```python
from build123d import *

# Parameters (mm, degrees)
SKETCH1_W           = 161.925
SKETCH1_H           = 152.4
SKETCH1_R           = 3.175
BOSS_EXTRUDE1_DEPTH = 12.7


with BuildPart() as part:
    # Sketch1 → Boss-Extrude1 (new body)
    with BuildSketch(Plane(origin=(0, 0, 0), x_dir=(0, 0, -1), z_dir=(1, 0, 0))):
        with Locations((20.6375, 0)):
            Rectangle(SKETCH1_W, SKETCH1_H)
        with Locations((95.25, -63.5)):
            Circle(SKETCH1_R, mode=Mode.SUBTRACT)
        with Locations((95.25, 0)):
            Circle(SKETCH1_R, mode=Mode.SUBTRACT)
        with Locations((-53.975, -63.5)):
            Circle(SKETCH1_R, mode=Mode.SUBTRACT)
        with Locations((-53.975, 0)):
            Circle(SKETCH1_R, mode=Mode.SUBTRACT)
        with Locations((95.25, 57.15)):
            Circle(SKETCH1_R, mode=Mode.SUBTRACT)
        with Locations((-53.975, 57.15)):
            Circle(SKETCH1_R, mode=Mode.SUBTRACT)
        with BuildLine():
            ThreePointArc((-33.455, 30.43), (-32.255, 29.23), (-33.455, 28.03))
            Line((-33.455, 28.03), (-36.055, 28.03))
            ThreePointArc((-36.055, 28.03), (-37.255, 29.23), (-36.055, 30.43))
            Line((-36.055, 30.43), (-33.455, 30.43))
        make_face(mode=Mode.SUBTRACT)
        with BuildLine():
            Line((-8.915, 28.03), (-11.515, 28.03))
            ThreePointArc((-11.515, 28.03), (-12.715, 29.23), (-11.515, 30.43))
            Line((-11.515, 30.43), (-8.915, 30.43))
            ThreePointArc((-8.915, 30.43), (-7.715, 29.23), (-8.915, 28.03))
        make_face(mode=Mode.SUBTRACT)
        with BuildLine():
            Line((-36.055, 48.17), (-33.455, 48.17))
            ThreePointArc((-33.455, 48.17), (-32.255, 46.97), (-33.455, 45.77))
            Line((-33.455, 45.77), (-36.055, 45.77))
            ThreePointArc((-36.055, 45.77), (-37.255, 46.97), (-36.055, 48.17))
        make_face(mode=Mode.SUBTRACT)
        with BuildLine():
            ThreePointArc((-8.915, 48.17), (-7.715, 46.97), (-8.915, 45.77))
            Line((-8.915, 45.77), (-11.515, 45.77))
            ThreePointArc((-11.515, 45.77), (-12.715, 46.97), (-11.515, 48.17))
            Line((-11.515, 48.17), (-8.915, 48.17))
        make_face(mode=Mode.SUBTRACT)
    extrude(amount=BOSS_EXTRUDE1_DEPTH)


solid = part.part
```
Design review of the part built by this model. Coordinates are the model's own, in mm. Coordinates: 2 decimals unless noted, no trailing zeros. Order: outer loops, then holes, each group sorted by start corner. A loop starts at its lowest first (then second) coordinate and runs counter-clockwise, first axis right, second up.
1) Take a section at A-A, the plane z = -95.25. Give the boundary of the cut face in (x, y) (3 decimals), and give its area (3 significant figures).
2) Take a section at B-B, the plane y = 57.15. Give the boundary of the cut face in (x, z) (3 decimals).
3) Wall thickness on line 1 along Y through (x, z) = (3.5, -95.25) (3 decimals): over which ranges is the line inside the solid? List them lowest first.
4) Clearance check with a flat-ended pin moving along its axis: pin 1 (5.5 mm diameter, centred on y = 0, z = -95.25, fed in from +X). State where the tip first meets the part, or that it passes through.
5) Mouldability with a two-part tool opening along Z and no side actions: class faces 1 (the flat face through (12.7, 1, -20)), 2 (the flat face through (6, -1, -101.6)), 3 (the cylindrical face through (6.261, 0.14, 57.147)) as +Z half, -Z half, draft (parallel to the pull), parting line (faces both ways), or undercut.
Returned:
1. outline: (0, -76.2) - (12.7, -76.2) - (12.7, -66.675) - (0, -66.675) - close; (0, -60.325) - (12.7, -60.325) - (12.7, -3.175) - (0, -3.175) - close; (0, 3.175) - (12.7, 3.175) - (12.7, 53.975) - (0, 53.975) - close; (0, 60.325) - (12.7, 60.325) - (12.7, 76.2) - (0, 76.2) - close
1. area: 1,690 mm2
2. outline: (0, -101.6) - (12.7, -101.6) - (12.7, -98.425) - (0, -98.425) - close; (0, -92.075) - (12.7, -92.075) - (12.7, 50.8) - (0, 50.8) - close; (0, 57.15) - (12.7, 57.15) - (12.7, 60.325) - (0, 60.325) - close
3. line 1: y = -76.2 to -66.675, -60.325 to -3.175, 3.175 to 53.975, 60.325 to 76.2
4. pin 1: passes through
5. face 1: draft
5. face 2: -Z half
5. face 3: undercut
